Input: dimensioned drawing with shaded views. Units: mm. Origin: part minimum x, y, z. A direction names the side the tool comes from. Coordinates: 2 decimals unless noted, no trailing zeros. Order: outer loops, then holes, each group sorted by start corner. A loop starts at its lowest first (then second) coordinate and runs counter-clockwise, first axis right, second up. Notation, with made-up numbers: (56.5, 84.25) - (104.5, 84.25) arc R10 ccw to (104.5, 95.25) - close; hole circle Ø9 at (77, 73). An arc over 180 degrees is marked (long way). Use one line per item in the form item = value. Start each with the question number.
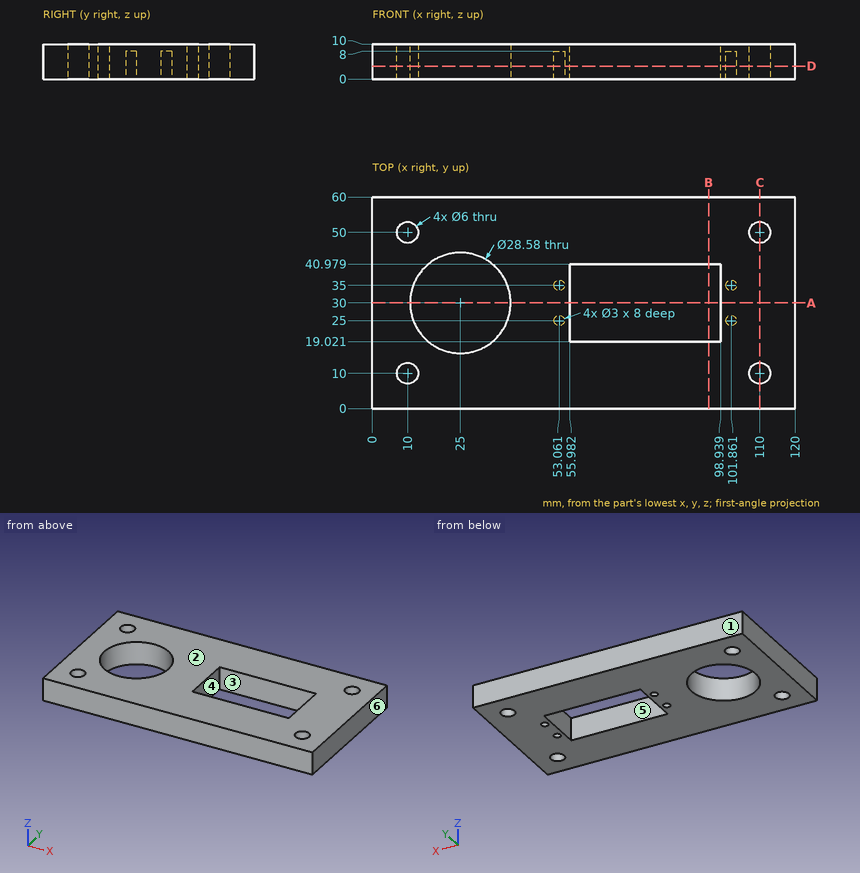
(1) Material intervals for L1, parallel to Y at x = 110, z = 7.25; L2, parallel to Y at x = 61, z = 8.75; L3, parallel to X at y = 22, z = 3.25, sorted ascending. Write a range as from..to.
(2) Set-up query: the marked faces 5 and 6. Return all of +Z, -Z, +X, -X, +Y, -Y with unobstructed straight access to the full face (end or side cutting, diameter ignored); none if empty.
(3) Contact query for flat-ended pins moving along their axis: pin 1 Ø3.5 at (x, y) = (101.86, 25) entering from -Z; pin 2 Ø5 at (x, y) = (110, 50) entering from +Z; pin 3 Ø0.9 at (x, y) = (53, 25.5) entering from -Z. Output: stop coordinate, or through.
(4) Cut plane D-D on z = 3.75. Count the separate pieces of the cut face and the enclosed holes in it, plus the area to 3 significant figures.
(5) Cut plane A-A on y = 30. Return the cut outline in (x, z).
(6) Cut plane C-C on x = 110. Return the cut outline in (y, z), plus the area to 3 significant figures.
(7) Cut plane B-B on x = 95.5. Return the cut outline in (y, z).
(8) Draft query along Y for the marked faces 1, 2, 3 and 4. Return one class per face: released by +Y, released by -Y, zero draft, split by the parting line, or undercut.
Check sheet entries:
q1.L1 = 0..7, 13..47, 53..60
q1.L2 = 0..19.02, 40.98..60
q1.L3 = 0..13.16, 36.84..55.98, 98.94..120
q2.face_5 = +Z, -Z
q2.face_6 = +Z, -Z, +X, +Y, -Y
q3.pin_1 = 0
q3.pin_2 = through
q3.pin_3 = 8
q4.separate_pieces = 1
q4.enclosed_holes = 10
q4.area = 5,470 mm^2
q5.outline = (0, 0) - (10.71, 0) - (10.71, 10) - (0, 10) - close; (39.29, 0) - (55.98, 0) - (55.98, 10) - (39.29, 10) - close; (98.94, 0) - (120, 0) - (120, 10) - (98.94, 10) - close
q6.outline = (0, 0) - (7, 0) - (7, 10) - (0, 10) - close; (13, 0) - (47, 0) - (47, 10) - (13, 10) - close; (53, 0) - (60, 0) - (60, 10) - (53, 10) - close
q6.area = 480 mm^2
q7.outline = (0, 0) - (19.02, 0) - (19.02, 10) - (0, 10) - close; (40.98, 0) - (60, 0) - (60, 10) - (40.98, 10) - close
q8.face_1 = released by +Y
q8.face_2 = zero draft
q8.face_3 = undercut
q8.face_4 = undercut
